Autodesk Inventor part; units mm, degrees
ref_plane "YZ Plane" through (0, 0, 0) normal (1, 0, 0) x (0, 1, 0)
ref_plane "XZ Plane" through (0, 0, 0) normal (0, 1, 0) x (-1, 0, 0)
ref_plane "XY Plane" through (0, 0, 0) normal (0, 0, 1) x (1, 0, 0)
sketch "Sketch1" plane through (0, 0, 0) normal (0, 0, 1) x (1, 0, 0)
  point P0 (0, 0)
sketch "Sketch2" plane through (0, 0, 0) normal (0, 0, 1) x (1, 0, 0)
  line L0 (-3.8935, 14.4789) -> (8.8065, 14.4789)
  line L1 (8.8065, 14.4789) -> (8.8065, -10.9211)
  line L2 (8.8065, -10.9211) -> (-3.8935, -10.9211)
  line L3 (-3.8935, 0) -> (-3.8935, 14.4789)
  line L4 (-3.8935, 0) -> (-22.9435, 0)
  line L5 (-22.9435, 0) -> (-22.9435, -10.9211)
  line L6 (-22.9435, -10.9211) -> (-3.8935, -10.9211)
  point P0 (0, 0)
  dimension "d1" = 25.4
extrude "Extrusion1" add sketch "Sketch2" along normal blind 19.05
fillet "Fillet1" radius 6.35 2 edges at (-22.9435, -5.4605, 0) (-22.9435, -5.4605, 19.05)
fillet "Fillet2" radius 3.175 1 edges at (-3.8935, 0, 9.525)
sketch "Sketch3" plane through (-22.9435, 0, 12.7) normal (0, 1, 0) x (1, 0, 0)
  circle A0 centre (9.525, 3.175) radius 4.7625
  line L0 (0, 6.35) -> (0, 0)
  line L1 (15.875, -6.35) -> (6.35, -6.35)
  point P0 (22.9435, 12.7)
  dimension "d7" = 9.525
  dimension "d8" = 9.525
  dimension "d9" = 9.525
extrude "Extrusion2" cut sketch "Sketch3" against normal through all
mirror "Mirror1" about plane through (8.8065, -10.9211, 0) normal (1, 0, 0)
properties part number "5.5bFeatureApplication"
Here's how the part is built. I have some questions about the finished solid (model axes, mm). A direction names the side the tool comes from. Coordinates: 2 decimals unless noted, no trailing zeros. Write each loop counter-clockwise with the first axis right and the second up, starting at its lowest first coordinate (ties: lowest second). Pieces come first, ordered by that corner, then holes. Notation, with made-up numbers: (74, -38.75) -> (127, -38.75) arc R20 ccw to (127, -12.75) -> close; hole circle Ø11 at (-32, 75). An arc over 180 degrees is marked (long way). Use a Markdown table: item, result. Add a question column.
(1) If we section it at B-B, the plane x = 28: Write out the boundary of the cut face in (y, z), and give its area (3 significant figures).
(2) We'd pull the mould along X, two halves only. Please class faces 1 (the flat face through (40.556, -6, 9)), 2 (the cylindrical face through (-21.133, -5.537, 1.91)), 3 (the flat face through (8, -1, 0)), 4 (the cylindrical face through (34.811, -5.384, 6.627)): +X half, -X half, draft (parallel to the pull), parting line (faces both ways), or undercut.
(3) For faces 5 (the flat face through (36, 0, 9)), 6 (the flat face through (8, -10.921, 9)), 7 (the flat face through (-18.4, 0, 9.4)), which set-ups out of +Z, -Z, +X, -X, +Y, -Y let a thin tool reach every point of the face, with its end or its side?
(4) I'm going to push flat-ended pins straight in: P1, Ø9, axis at y = 9.5, z = 13, coming from the -X side; P2, Ø3, axis at x = -15.5, y = 2.5, coming from the -Z side; P3, Ø5, axis at x = 24.5, z = 6, coming from the +Y side; P4, Ø5.5, axis at y = 11.5, z = 14, coming from the +X side. Where does each tip first touch, or does it pass through?
(5) If we section it at A-A, the plane z = 8: State how many separate pieces and enclosed holes the cut face has, and give its area (3 significant figures).
(6) Please list where these lines run through material, in increasing order: line 1 (X direction, y = -5.5, z = 9.5); line 2 (X direction, y = -1.5, z = 8); line 3 (X direction, y = 9.5, z = 18).
Outcome:
| question | item | result |
|---|---|---|
| 1 | outline | (-10.92, 0) -> (0, 0) -> (0, 5.85) -> (-10.92, 5.85) -> close; (-10.92, 13.2) -> (0, 13.2) -> (0, 19.05) -> (-10.92, 19.05) -> close |
| 1 | area | 128 mm^2 |
| 2 | face 1 | +X half |
| 2 | face 2 | -X half |
| 2 | face 3 | draft |
| 2 | face 4 | undercut |
| 3 | face 5 | +Z, -Z, +X, +Y |
| 3 | face 6 | +Z, -Z, +X, -X, -Y |
| 3 | face 7 | +Z, -Z, -X, +Y |
| 4 | P1 | stops at x = -3.89 |
| 4 | P2 | passes through |
| 4 | P3 | stops at y = 1.47 |
| 4 | P4 | stops at x = 21.51 |
| 5 | separate pieces | 3 |
| 5 | enclosed holes | 0 |
| 5 | area | 868 mm^2 |
| 6 | line 1 | x = -22.94 to -18.18, -8.66 to 26.27, 35.79 to 40.56 |
| 6 | line 2 | x = -22.94 to -17.93, -8.91 to 26.52, 35.54 to 40.56 |
| 6 | line 3 | x = -3.89 to 21.51 |
